Design review of the part built by this model. Coordinates are the model's own, in mm. Face numbers are marked on the shaded views. A direction names the side the tool comes from. Coordinates: 2 decimals unless noted, no trailing zeros. Loops run counter-clockwise (first coordinate to the right, second up) from the corner with the lowest first, then second, coordinate; pieces in that order, holes last. Notation, with made-up numbers: M 80.5,63 L 121.5,63 A35 ccw 121.5,96 Z; hole C -10,-0.75 d7. An arc over 180 degrees is marked long. Answer as a JSON object with one key per item and string values. Group by question number.
1. Machinability: for the marked faces 1, 2 and 3, which of the approach directions +Z, -Z, +X, -X, +Y, -Y give a long, thin tool a straight path to every point of the face, cutting with its end or side? Answer none if there is none.
2. Consider section C-C (z = -12). Count the separate pieces of the cut face and the enclosed holes in it, then the cut area to 3 significant figures.
3. To check wall thickness, follow probe 1 along X at (y, z) = (36.85, 0); probe 2 along X at (y, z) = (36, 0). State the ranges of each line that lie inside material, in increasing order.
4. Draft analysis for pull direction Z (two halves, no side actions). For the marked faces 4, 5 and 6, state which applies: +Z half, -Z half, draft (parallel to the pull), parting line (faces both ways), or undercut.
5. Insertion check: pin 1 (7 mm diameter, centred on x = -13.44, z = 13.44, fed in from -Y); pin 2 (5 mm diameter, centred on x = 13.44, z = -13.44, fed in from +Y); pin 3 (3 mm diameter, centred on y = 19, z = -8.5, fed in from -X). Each pin has a flat end and moves straight along its axis. Give the tip position at first contact, or say it passes through.
6. Consider section A-A (y = 21). State the section outline as (x, z) points, then the cut area to 3 significant figures.
7. Consider section B-B (y = 3). State the section outline as (x, z) points.
from build123d import *

# Parameters (mm, degrees)
FLANGE_DEPTH         = 6
SKETCH9_R            = 4
COUNTERBORE_DEPTH    = 4.1
SKETCH10_R           = 2.25
MOUNTING_HOLES_DEPTH = 33.9
SKETCH11_R           = 0.375
CHAMFER1_SIZE        = 0.2


with BuildPart() as part:
    # Sketch5 → Bearing Body (revolve)
    with BuildSketch(Plane(origin=(0, 0, 0), x_dir=(0, 0, -1), z_dir=(1, 0, 0))):
        Polygon((8.5, 37), (8, 37), (8, 0), (8.5, 0), (8.5, 0.8), (13.5, 0.8), (13.5, 0), (14, 0), (14, 37), (13.5, 37), (13.5, 36.2), (8.5, 36.2), align=None)
    revolve(axis=Axis((0, 0, 0), (0, 1, 0)))

    # Sketch8 → Flange (add)
    with BuildSketch(Plane(origin=(0, 0, 0), x_dir=(1, 0, 0), z_dir=(0, 1, 0))):
        Polygon((0, -18.5), (-16.5, -18.5), (-18.5, -16.5), (-18.5, 0), (-18.5, 16.5), (-16.5, 18.5), (0, 18.5), (16.5, 18.5), (18.5, 16.5), (18.5, 0), (18.5, -16.5), (16.5, -18.5), align=None)
        with BuildLine():
            ThreePointArc((-10.5, 0), (-7.424621202, -7.424621202), (0, -10.5))
            ThreePointArc((0, -10.5), (7.424621202, -7.424621202), (10.5, 0))
            ThreePointArc((10.5, 0), (7.424621202, 7.424621202), (0, 10.5))
            ThreePointArc((0, 10.5), (-7.424621202, 7.424621202), (-10.5, 0))
        make_face(mode=Mode.SUBTRACT)
    extrude(amount=FLANGE_DEPTH)

    # Sketch9 → Counterbore (cut)
    with BuildSketch(Plane(origin=(0, 0, 0), x_dir=(-1, 0, 0), z_dir=(0, -1, 0))):
        with Locations((13.435028843, -13.435028843)):
            Circle(SKETCH9_R)
        with Locations((-13.435028843, -13.435028843)):
            Circle(SKETCH9_R)
        with Locations((-13.435028843, 13.435028843)):
            Circle(SKETCH9_R)
        with Locations((13.435028843, 13.435028843)):
            Circle(SKETCH9_R)
    extrude(amount=-COUNTERBORE_DEPTH, mode=Mode.SUBTRACT)

    # Sketch10 → Mounting Holes (cut, through all)
    with BuildSketch(Plane(origin=(0, 4.1, 0), x_dir=(-1, 0, 0), z_dir=(0, -1, 0))):
        with Locations((13.435028843, 13.435028843)):
            Circle(SKETCH10_R)
        with Locations((13.435028843, -13.435028843)):
            Circle(SKETCH10_R)
        with Locations((-13.435028843, -13.435028843)):
            Circle(SKETCH10_R)
        with Locations((-13.435028843, 13.435028843)):
            Circle(SKETCH10_R)
    extrude(amount=-MOUNTING_HOLES_DEPTH, mode=Mode.SUBTRACT)

    # Sketch11 → Relief (revolve, cut)
    with BuildSketch(Plane(origin=(0, 0, 0), x_dir=(0, 0, -1), z_dir=(1, 0, 0))):
        with Locations((-14.026134699, 6)):
            Circle(SKETCH11_R)
    revolve(axis=Axis((0, 0, 0), (0, 1, 0)), mode=Mode.SUBTRACT)

    # Chamfer1
    chamfer1_edges = [part.edges().sort_by_distance(p)[0] for p in [
        (-17.5, 6, 17.5),
        (0, 6, 18.5),
        (17.5, 6, 17.5),
        (18.5, 6, 0),
        (17.5, 6, -17.5),
        (0, 6, -18.5),
        (-17.5, 6, -17.5),
        (-18.5, 6, 0),
        (-17.5, 0, 17.5),
        (0, 0, 18.5),
        (17.5, 0, 17.5),
        (18.5, 0, 0),
        (17.5, 0, -17.5),
        (0, 0, -18.5),
        (-17.5, 0, -17.5),
        (-18.5, 0, 0),
    ]]
    chamfer(chamfer1_edges, length=CHAMFER1_SIZE)


solid = part.part
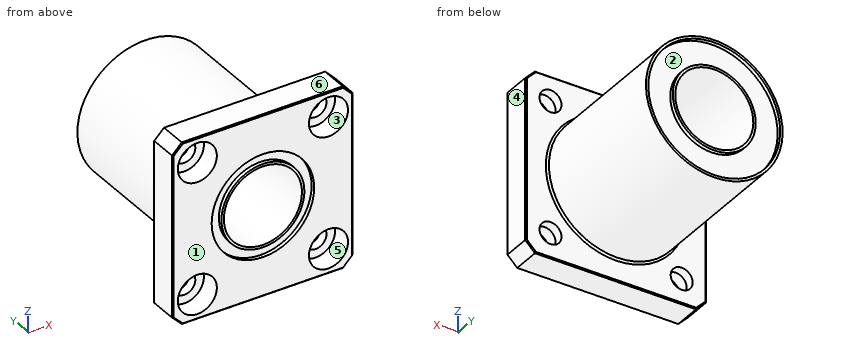
Findings below:
{
 "1": {"face 1": "+Z, -Z, +X, -X, -Y", "face 2": "+Y", "face 3": "-Y"},
 "2": {"separate pieces": "3", "enclosed holes": "0", "area": "583 mm^2"},
 "3": {"probe 1": "x = -14 to -13.5, -8.5 to -8, 8 to 8.5, 13.5 to 14", "probe 2": "x = -14 to -8, 8 to 14"},
 "4": {"face 4": "draft", "face 5": "undercut", "face 6": "+Z half"},
 "5": {"pin 1": "stops at y = 4.1", "pin 2": "stops at y = 6", "pin 3": "stops at x = -12.12"},
 "6": {"outline": "C 0,0 d28; hole C 0,0 d16", "area": "415 mm^2"},
 "7": {"outline": "M -18.5,-16.5 L -16.5,-18.5 L 16.5,-18.5 L 18.5,-16.5 L 18.5,16.5 L 16.5,18.5 L -16.5,18.5 L -18.5,16.5 Z; hole C -13.44,-13.44 d8; hole C -13.44,13.44 d8; hole C 0,0 d16; hole C 13.44,-13.44 d8; hole C 13.44,13.44 d8"}
}
